For this review, take the finished solid that the model builds, in its own axes (mm). A direction names the side the tool comes from. Round coordinates to 2 decimals unless told otherwise and drop trailing zeros. Write each loop counter-clockwise with the first axis right and the second up, starting at its lowest first coordinate (ties: lowest second). Pieces come first, ordered by that corner, then holes. Notation, with made-up numbers: M 65,-35 L 117,-35 A9 ccw 117,-27 Z; hole C 54.5,-30.5 d8. An arc over 180 degrees is marked long. Use one line per item in the form item = value. Start each with the question number.
Item 1: For faces 1 (the cylindrical face through (22.6, -8.78, 13.35)), 2 (the flat face through (64, 0, -5.55)), 3 (the flat face through (59, 0, -12.7)), 4 (the cylindrical face through (21.199, -26.054, 6.676)), 5 (the flat face through (10, 0, -10)), list the 3-axis set-ups (+Z, -Z, +X, -X, +Y, -Y) from which the entire face can be reached by the end or side of a thin tool; tool diameter is ignored.
Item 2: Add section D-D (z = -18.5). State the section outline as (x, y) points.
Item 3: For P1, Ø5, axis at y = -15, z = -17, coming from the +X side; P2, Ø4, axis at x = 72, y = 9, coming from the +Z side; P3, Ø10, axis at y = -15, z = 5, coming from the -X side, all flat-tipped, find the tip position at first contact; note any pin that passes through.
Item 4: Add section A-A (z = 50.8). State the section outline as (x, y) points, and give its area (3 significant figures).
Item 5: Add section C-C (y = -14.5). State the section outline as (x, z) points, and give its area (3 significant figures).
Item 6: Add section B-B (x = 7). State the section outline as (y, z) points, and give its area (3 significant figures).
Item 7: For line 1 (Z direction, x = 0, y = 13) (3 decimals); line 2 (Y direction, x = 83, z = 7), list the stretches that pass through material, from the lowest coordinate up. Write a range as [from, to].
Item 8: Draft analysis for pull direction X (two halves, no side actions). For faces 6 (the cylindrical face through (99.4, -0.2, 56.4)), 7 (the cylindrical face through (126.184, -0.178, 14.376)), 8 (the cylindrical face through (90.254, -8.78, 47.059)), state which applies: released by +X, released by -X, zero draft, split by the parting line, or undercut.
from build123d import *

# Parameters (mm, degrees)
F0_R     = 22.225
F1_DEPTH = 35.7124
F2_DEPTH = 16.6624
F3_DEPTH = 4.7625
F4_DEPTH = 12.6873


with BuildPart() as f1:
    # F0 (on Front) → F1 (new body)
    with BuildSketch(Plane.XZ):
        Circle(F0_R)
        with BuildLine():
            ThreePointArc((0, 12.7), (8.980256, 8.980256), (12.7, 0))
            ThreePointArc((12.7, 0), (8.980256, -8.980256), (0, -12.7))
            ThreePointArc((0, -12.7), (-12.7, 0), (0, 12.7))
        make_face(mode=Mode.SUBTRACT)
    extrude(amount=F1_DEPTH)

    # F0 (on Front) → F2 (join, symmetric)
    with BuildSketch(Plane.XZ):
        with BuildLine():
            ThreePointArc((20.32, -15.24), (24.096556, -8.032185), (25.4, 0))
            ThreePointArc((25.4, 0), (24.096556, 8.032185), (20.32, 15.24))
            ThreePointArc((20.32, 15.24), (11.359225, 22.718451), (0, 25.4))
            ThreePointArc((0, 25.4), (-22.718451, -11.359225), (20.32, -15.24))
        make_face()
        Circle(F0_R, mode=Mode.SUBTRACT)
    extrude(amount=F2_DEPTH, both=True)

    # F0 (on Front) → F3 (join, symmetric)
    with BuildSketch(Plane.XZ):
        with BuildLine():
            ThreePointArc((0, 25.4), (11.359225, 22.718451), (20.32, 15.24))
            ThreePointArc((20.32, 15.24), (22.560194, 13.370387), (25.4, 12.7))
            Line((25.4, 12.7), (93.325559, 12.7))
            ThreePointArc((93.325559, 12.7), (98.244248, 15.033907), (99.547263, 20.32))
            ThreePointArc((99.547263, 20.32), (96.086385, 33.014641), (91.013932, 45.155556))
            ThreePointArc((91.013932, 45.155556), (90.262515, 47.032005), (89.818321, 49.003903))
            ThreePointArc((89.818321, 49.003903), (88.705969, 44.424273), (84.743782, 41.872523))
            Line((84.743782, 41.872523), (0, 25.4))
        make_face()
    extrude(amount=F3_DEPTH, both=True)

    # F0 (on Front) → F4 (join, symmetric)
    with BuildSketch(Plane.XZ):
        with BuildLine():
            ThreePointArc((20.32, 15.24), (24.096556, 8.032185), (25.4, 0))
            ThreePointArc((25.4, 0), (24.096556, -8.032185), (20.32, -15.24))
            ThreePointArc((20.32, -15.24), (22.560194, -13.370387), (25.4, -12.7))
            Line((25.4, -12.7), (93.325559, -12.7))
            ThreePointArc((93.325559, -12.7), (98.244248, -15.033907), (99.547263, -20.32))
            ThreePointArc((99.547263, -20.32), (99.309847, -21.450275), (99.059598, -22.577778))
            ThreePointArc((99.059598, -22.577778), (108.619825, -37.78245), (123.824497, -28.222222))
            ThreePointArc((123.824497, -28.222222), (126.113403, 14.98031), (113.767415, 56.444444))
            ThreePointArc((113.767415, 56.444444), (98.622679, 62.928158), (89.818321, 49.003903))
            ThreePointArc((89.818321, 49.003903), (90.262515, 47.032005), (91.013932, 45.155556))
            ThreePointArc((91.013932, 45.155556), (96.086385, 33.014641), (99.547263, 20.32))
            ThreePointArc((99.547263, 20.32), (98.244248, 15.033907), (93.325559, 12.7))
            Line((93.325559, 12.7), (25.4, 12.7))
            ThreePointArc((25.4, 12.7), (22.560194, 13.370387), (20.32, 15.24))
        make_face()
        with BuildLine():
            ThreePointArc((44.45, -5.5499), (38.9001, 0), (44.45, 5.5499))
            Line((44.45, 5.5499), (82.55, 5.5499))
            ThreePointArc((82.55, 5.5499), (88.0999, 0), (82.55, -5.5499))
            Line((82.55, -5.5499), (44.45, -5.5499))
        make_face(mode=Mode.SUBTRACT)
        with BuildLine():
            ThreePointArc((96.702303, 47.977778), (99.568451, 56.488371), (108.079044, 53.622222))
            ThreePointArc((108.079044, 53.622222), (119.807732, 14.231294), (117.633273, -26.811111))
            ThreePointArc((117.633273, -26.811111), (110.030937, -31.591225), (105.250823, -23.988889))
            ThreePointArc((105.250823, -23.988889), (107.196392, 12.733263), (96.702303, 47.977778))
        make_face(mode=Mode.SUBTRACT)
    extrude(amount=F4_DEPTH, both=True)


solid = f1.part
Calculated:
q1.face_1 = +Z, -Y
q1.face_2 = +Y, -Y
q1.face_3 = -Z, +Y, -Y
q1.face_4 = -Y
q1.face_5 = +Y
q2.outline = M -17.4,-16.66 L -12.32,-16.66 L -12.32,-35.71 L 12.32,-35.71 L 12.32,-16.66 L 17.4,-16.66 L 17.4,16.66 L 12.32,16.66 L 12.32,0 L -12.32,0 L -12.32,16.66 L -17.4,16.66 Z; M 99.65,-12.69 L 106.35,-12.69 L 106.35,12.69 L 99.65,12.69 Z; M 119.22,-12.69 L 125.65,-12.69 L 125.65,12.69 L 119.22,12.69 Z
q3.P1 = 125.98
q3.P2 = 12.7
q3.P3 = -25.4
q4.outline = M 89.69,-12.69 L 96.04,-12.69 L 96.04,12.69 L 89.69,12.69 Z; M 109.43,-12.69 L 116.4,-12.69 L 116.4,12.69 L 109.43,12.69 Z
q4.area = 338 mm^2
q5.outline = M 0,25.4 A25.4 ccw long 20.32,-15.24 A25.4 ccw 25.4,0 A25.4 ccw 20.32,15.24 A25.4 ccw Z; hole C 0,0 d25.4
q5.area = 1,520 mm^2
q6.outline = M -35.71,-21.09 L -16.66,-21.09 L -16.66,-24.42 L 16.66,-24.42 L 16.66,-21.09 L 0,-21.09 L 0,-10.6 L -35.71,-10.6 Z; M -35.71,10.6 L 0,10.6 L 0,21.09 L 16.66,21.09 L 16.66,24.42 L 4.76,24.42 L 4.76,26.76 L -4.76,26.76 L -4.76,24.42 L -16.66,24.42 L -16.66,21.09 L -35.71,21.09 Z
q6.area = 994 mm^2
q7.line_1 = [-25.4, -22.225], [22.225, 25.4]
q7.line_2 = [-12.69, 12.69]
q8.face_6 = undercut
q8.face_7 = released by +X
q8.face_8 = released by -X
